The model under review builds one solid part; all positions refer to its coordinate system, in mm. Coordinates: 2 decimals unless noted, no trailing zeros. Order: outer loops, then holes, each group sorted by start corner. A loop starts at its lowest first (then second) coordinate and runs counter-clockwise, first axis right, second up. Notation, with made-up numbers: (54, 17) - (84, 17) arc R24 cw to (84, 39) - close; hole circle Ø8 at (62.5, 43). An arc over 180 degrees is marked (long way). Answer in a Markdown table with one row per item.
Autodesk Inventor part; units mm, degrees
ref_plane "YZ Plane" through (0, 0, 0) normal (1, 0, 0) x (0, 1, 0)
ref_plane "XZ Plane" through (0, 0, 0) normal (0, 1, 0) x (-1, 0, 0)
ref_plane "XY Plane" through (0, 0, 0) normal (0, 0, 1) x (1, 0, 0)
sketch "Esboço1" plane through (0, 0, 0) normal (1, 0, 0) x (0, 1, 0)
  line L0 (0, 0) -> (50.8, 0)
  line L1 (50.8, 0) -> (50.8, -86.2)
  line L2 (50.8, -86.2) -> (0, -86.2)
  line L3 (0, -86.2) -> (0, 0)
  dimension "d0" = 50.8
  dimension "d1" = 86.2
extrude "Extrusão1" add sketch "Esboço1" along normal blind 5
sketch "Esboço2" plane through (5, 0, 0) normal (1, 0, 0) x (0, 0, -1)
  circle A0 centre (5, 12.7) radius 2.5
  circle A1 centre (5, 25.4) radius 2.5
  circle A2 centre (5, 38.1) radius 2.5
  line L0 (0, 50.8) -> (0, 0)
  line L1 (86.2, 50.8) -> (0, 50.8)
  line L2 (0, 0) -> (86.2, 0)
  dimension "d4" = 5
  dimension "d5" = 5
  dimension "d6" = 5
  dimension "d7" = 5
  dimension "d8" = 5
  dimension "d9" = 5
  dimension "d10" = 12.7
  dimension "d11" = 12.7
  dimension "d12" = 12.7
extrude "Extrusão2" cut sketch "Esboço2" against normal blind 6
pattern_linear "Padrão retangular1" count 7 spacing 12.7 along (0, 0, -1) of "Extrusão2"
sketch "Esboço3" plane through (0, 0, 0) normal (-1, 0, 0) x (0, 0, 1)
  line L0 (0, 50.8) -> (0, 0)
  line L1 (0, 0) -> (-86.2, 0)
  line L2 (0, 50.8) -> (-50.8, 50.8)
  line L3 (-50.8, 50.8) -> (-50.8, 0)
  line L4 (-50.8, 0) -> (0, 0)
  line L5 (0, 0) -> (0, 50.8)
  circle A0 centre (-55.8, 25.4) radius 2.5
  dimension "d19" = 5
extrude "Extrusão3" cut sketch "Esboço3" against normal blind 10 contours L0 L1 L3 L2
sketch "Esboço4" plane through (5, 0, 0) normal (1, 0, 0) x (0, 0, -1)
  line L0 (86.2, 0) -> (86.2, 50.8)
  line L1 (86.2, 50.8) -> (124.3, 50.8)
  line L2 (124.3, 50.8) -> (124.3, 0)
  line L3 (124.3, 0) -> (86.2, 0)
  line L4 (86.2, 0) -> (86.2, 50.8)
  circle A0 centre (93.9, 25.4) radius 2.5
  circle A1 centre (93.9, 38.1) radius 2.5
  circle A2 centre (106.6, 38.1) radius 2.5
  circle A3 centre (119.3, 38.1) radius 2.5
  circle A4 centre (119.3, 25.4) radius 2.5
  circle A5 centre (106.6, 25.4) radius 2.5
  circle A6 centre (93.9, 12.7) radius 2.5
  circle A7 centre (106.6, 12.7) radius 2.5
  circle A8 centre (119.3, 12.7) radius 2.5
  point P0 (0, 0)
  dimension "d22" = 5
  dimension "d23" = 50.8
extrude "Extrusão4" add sketch "Esboço4" against normal blind 5
sketch "Esboço7" plane through (5, 0, 0) normal (1, 0, 0) x (0, 0, -1)
  line L0 (124.3, 50.8) -> (50.8, 50.8)
  line L1 (124.3, 50.8) -> (124.3, 85.9607)
  circle A0 centre (95.7, 85.9607) radius 11.25
  circle A1 centre (-89.125, 144.496) radius 17.5
  circle A2 centre (95.7, 111.3607) radius 2.0193
  circle A3 centre (77.7395, 103.9212) radius 2.0193
  circle A4 centre (95.7, 60.5607) radius 2.0193
  circle A5 centre (113.6605, 68.0002) radius 2.0193
  circle A6 centre (-101.825, 169.896) radius 2.5
  circle A7 centre (-76.425, 169.896) radius 2.5
  circle A8 centre (-76.425, 119.096) radius 2.5
  circle A9 centre (-101.825, 119.096) radius 2.5
  arc A10 (-76.1735, 179.6885) -> (-105.0332, 110.5375) centre (-89.125, 144.496) ccw
  arc A11 (124.3, 85.9607) -> (105.5776, 112.8008) centre (95.7, 85.9607) ccw
  line L2 (50.8, 0) -> (50.8, 50.8)
  line L3 (50.8, 50.8) -> (50.8, 110.5375)
  line L4 (50.8, 110.5375) -> (-105.0332, 110.5375)
  line L5 (54.784, 109.5375) -> (24.05, 109.5375)
  line L6 (-76.1735, 179.6885) -> (105.5776, 112.8008)
  circle A12 centre (-89.125, 144.496) radius 20
  circle A13 centre (95.7, 85.9607) radius 14.25
  point P0 (0, 0)
  dimension "d36" = 75
  dimension "d37" = 1
  dimension "d38" = 40
  dimension "d39" = 28.5
extrude "Extrusão6" add sketch "Esboço7" against normal blind 5 contours L0 L3 L4 A10 L6 A11 L1
fillet "Arredondamento1" radius 5 4 edges at (2.5, 110.5375, -50.8) (2.5, 110.5375, 105.0332) (2.5, 0, -50.8) (2.5, 0, -124.3)
sketch "Esboço8" plane through (5, 0, 0) normal (1, 0, 0) x (0, 0, -1)
  circle A0 centre (-2.9415, 147.4099) radius 2.5
  point P0 (0, 0)
extrude "Extrusão7" cut sketch "Esboço8" against normal blind 10
equation "\"d8\" = d7"
equation "\"d9\" = d8"
equation "\"d11\" = d10"
equation "\"d12\" = d11"
properties part number "CHAPA FIXAÇÃO ESQUERDA 2"
Item 1: We need section A-A, the plane z = -68.5. Write out the cut boundary in (x, y), then the cut area to 3 significant figures.
Check values:
| item | result |
|---|---|
| outline | (0, 0) - (5, 0) - (5, 10.2) - (0, 10.2) - close; (0, 15.2) - (5, 15.2) - (5, 22.9) - (0, 22.9) - close; (0, 27.9) - (5, 27.9) - (5, 35.6) - (0, 35.6) - close; (0, 40.6) - (5, 40.6) - (5, 126.45) - (0, 126.45) - close |
| area | 557 mm^2 |
Item 2: To check wall thickness, follow line 1 (Z direction, x = 3.3, y = 44); line 2 (Y direction, x = 2.9, z = -81.2); line 3 (Z direction, x = 2.15, y = 88). State the ranges of each line that lie inside material, in increasing order. Write a range as from..to.
Check values:
| item | result |
|---|---|
| line 1 | -124.3..-50.8 |
| line 2 | 0..10.2, 15.2..22.9, 27.9..35.6, 40.6..121.77 |
| line 3 | -124.23..-109.8, -81.6..-50.8 |
Item 3: Mouldability with a two-part tool opening along Y and no side actions: class faces 1 (the face through (2.535, 13.451, -83.585)), 2 (the face through (0, 112, -25)), 3 (the face through (2.46, 1.5, -122.87)) as +Y half, -Y half, draft (parallel to the pull), parting line (faces both ways), or undercut.
Check values:
| item | result |
|---|---|
| face 1 | undercut |
| face 2 | draft |
| face 3 | -Y half |
Item 4: We need section C-C, the plane y = 135.5. Write out the cut boundary in (x, z).
Check values:
| item | result |
|---|---|
| outline | (0, -43.9) - (5, -43.9) - (5, 71.26) - (0, 71.26) - close; (0, 106.99) - (5, 106.99) - (5, 125.53) - (0, 125.53) - close |
Item 5: Clearance check with flat-ended pins moving along their axes: pin 1 Ø6.5 at (y, z) = (60.56, -95.7) entering from -X; pin 2 Ø2.5 at (x, z) = (1.5, 38.5) entering from -Y; pin 3 Ø1.5 at (x, z) = (3, -78.5) entering from +Y; pin 4 Ø1.5 at (x, z) = (3.5, 92) entering from +Y. State where each tip first meets the part, or that it passes through.
Check values:
| item | result |
|---|---|
| pin 1 | x = 0 |
| pin 2 | y = 110.54 |
| pin 3 | y = 123.04 |
| pin 4 | y = 181.94 |
Item 6: We need section D-D, the plane x = 2.6. State how many separate pieces and enclosed holes the cut face has, then the cut area to 3 significant figures.
Check values:
| item | result |
|---|---|
| separate pieces | 1 |
| enclosed holes | 29 |
| area | 15,200 mm^2 |
Item 7: We need section B-B, the plane y = 162. Write out the cut boundary in (x, z), then the cut area to 3 significant figures.
Check values:
| item | result |
|---|---|
| outline | (0, 28.11) - (5, 28.11) - (5, 79.45) - (0, 79.45) - close; (0, 98.8) - (5, 98.8) - (5, 122.29) - (0, 122.29) - close |
| area | 374 mm^2 |
